from build123d import *

# Parameters (mm, degrees)
SKETCH1_W           = 15.875
SKETCH1_H           = 11.239799379
BOSS_EXTRUDE1_DEPTH = 2.54
BOSS_EXTRUDE2_REACH = 31.638
SKETCH2_W           = 1.27
SKETCH2_H           = 5.08
SKETCH2_W_2         = 3.81
SKETCH2_H_2         = 1.624267758
BOSS_EXTRUDE3_REACH = 23.94
FILLET1_R           = 0.127


with BuildPart() as part:
    # Sketch1 → Boss-Extrude1 (new body)
    with BuildSketch(Plane.XY):
        with Locations((7.9375, -19.278367991)):
            Rectangle(SKETCH1_W, SKETCH1_H)
    extrude(amount=BOSS_EXTRUDE1_DEPTH)

    # Boss-Extrude2: up to this plane
    boss_extrude2_end = Plane(origin=(1.6499976, -12.666472126, 11.206213123), z_dir=(-1.2251589112771177e-15, 0.017452406437284806, -0.9998476951563913))
    # Sketch2 → Boss-Extrude2 (add, up to the surface)
    with BuildSketch(Plane.XY.offset(2.54), mode=Mode.PRIVATE) as boss_extrude2_sk1:
        with BuildLine():
            Line((2.625, -17.673999922), (2.625, -19.753999922))
            Line((2.625, -19.753999922), (1.355, -19.753999922))
            Line((1.355, -19.753999922), (1.355, -14.673999922))
            Line((1.355, -14.673999922), (2.625, -14.673999922))
            Line((2.625, -14.673999922), (2.625, -17.273999922))
            Line((2.625, -17.273999922), (2.375, -17.273999922))
            Line((2.375, -17.273999922), (2.375, -17.473999922))
            ThreePointArc((2.375, -17.473999922), (2.433578644, -17.615421279), (2.575, -17.673999922))
            Line((2.575, -17.673999922), (2.625, -17.673999922))
        make_face()
    boss_extrude2_tool1 = split(extrude(boss_extrude2_sk1.sketch, amount=BOSS_EXTRUDE2_REACH, mode=Mode.PRIVATE), bisect_by=boss_extrude2_end, keep=Keep.BOTH, mode=Mode.PRIVATE)
    add(boss_extrude2_tool1.solids().sort_by_distance((1.982561, -17.210473, 2.54))[0])
    # Sketch2 → Boss-Extrude2 (add, up to the surface)
    with BuildSketch(Plane.XY.offset(2.54), mode=Mode.PRIVATE) as boss_extrude2_sk2:
        with Locations((10.26, -17.213999922)):
            Rectangle(SKETCH2_W, SKETCH2_H)
    boss_extrude2_tool2 = split(extrude(boss_extrude2_sk2.sketch, amount=BOSS_EXTRUDE2_REACH, mode=Mode.PRIVATE), bisect_by=boss_extrude2_end, keep=Keep.BOTH, mode=Mode.PRIVATE)
    add(boss_extrude2_tool2.solids().sort_by_distance((10.26, -17.214, 2.54))[0])
    # Sketch2 → Boss-Extrude2 (add, up to the surface)
    with BuildSketch(Plane.XY.offset(2.54), mode=Mode.PRIVATE) as boss_extrude2_sk3:
        with Locations((6.375, -24.086133801)):
            Rectangle(SKETCH2_W_2, SKETCH2_H_2)
    boss_extrude2_tool3 = split(extrude(boss_extrude2_sk3.sketch, amount=BOSS_EXTRUDE2_REACH, mode=Mode.PRIVATE), bisect_by=boss_extrude2_end, keep=Keep.BOTH, mode=Mode.PRIVATE)
    add(boss_extrude2_tool3.solids().sort_by_distance((6.375, -24.086134, 2.54))[0])

    # Boss-Extrude3: up to this face of the body (flat: up to its plane)
    boss_extrude3_end = Plane(part.part.faces().sort_by_distance((1.99, -19.753999922, 6.811249933))[0])
    # Sketch4 → Boss-Extrude3 (add, up to the picked face)
    with BuildSketch(Plane.XZ.offset(14.673999922), mode=Mode.PRIVATE) as boss_extrude3_sk1:
        Polygon((10.895, 11.082499866), (9.625, 11.082499866), (9.625, 10.790559516), (8.992585474, 11.181716662), (10.895, 14.257499866), align=None)
    boss_extrude3_tool1 = split(extrude(boss_extrude3_sk1.sketch, amount=BOSS_EXTRUDE3_REACH, mode=Mode.PRIVATE), bisect_by=boss_extrude3_end, keep=Keep.BOTH, mode=Mode.PRIVATE)
    # Sketch4 → Boss-Extrude3 (add, up to the picked face)
    with BuildSketch(Plane.XZ.offset(14.673999922), mode=Mode.PRIVATE) as boss_extrude3_sk2:
        Polygon((1.355, 11.082499866), (2.625, 11.082499866), (2.625, 10.790559516), (3.26, 11.082499866), (1.355, 14.257499866), align=None)
    boss_extrude3_tool2 = split(extrude(boss_extrude3_sk2.sketch, amount=BOSS_EXTRUDE3_REACH, mode=Mode.PRIVATE), bisect_by=boss_extrude3_end, keep=Keep.BOTH, mode=Mode.PRIVATE)
    add(boss_extrude3_tool1.solids().sort_by(Axis((10.227849, -14.674, 12.119311), (0, -1, 0)))[0])
    add(boss_extrude3_tool2.solids().sort_by(Axis((2.015179, -14.674, 12.106466), (0, -1, 0)))[0])

    # Fillet1
    fillet1_edges = [part.edges().sort_by_distance(p)[0] for p in [
        (10.895, -14.673999922, 8.398749933),
        (10.895, -19.753999922, 8.398749933),
        (1.355, -19.753999922, 8.398749933),
        (1.355, -14.673999922, 8.398749933),
        (6.375, -23.273999922, 11.021058037),
        (8.28, -24.086133801, 11.006882187),
        (6.375, -24.89826768, 10.992706338),
        (4.47, -24.086133801, 11.006882187),
        (8.992585474, -17.213999922, 11.181716662),
        (10.895, -17.213999922, 14.257499866),
        (1.355, -17.213999922, 14.257499866),
        (3.26, -17.213999922, 11.082499866),
    ]]
    fillet(fillet1_edges, radius=FILLET1_R)


solid = part.part
Input: part model. Units: mm. Frame: model coordinates. A direction names the side the tool comes from. Round coordinates to 2 decimals unless told otherwise and drop trailing zeros. Order: outer loops, then holes, each group sorted by start corner. A loop starts at its lowest first (then second) coordinate and runs counter-clockwise, first axis right, second up. Notation, with made-up numbers: (51.5, 54.25) - (63.5, 54.25) arc R15 cw to (63.5, 77.25) - close; hole circle Ø5 at (88.25, 73). An arc over 180 degrees is marked (long way). Answer as a JSON object with one key per item and string values. Group by question number.
(1) Cut plane B-B (x = 6.5). Return loops of the section in (y, z), then the cut area to 3 significant figures.
(2) Pin query (flat end, axial travel): P1, Ø1.9, axis at x = 10, z = 7, coming from the -Y side; P2, Ø3, axis at y = -23, z = 3.5, coming from the +X side (3 decimals); P3, Ø1.9, axis at x = 2.5, z = 9.5, coming from the +Y side; P4, Ø1.5, axis at y = -17, z = 10.5, coming from the +X side (3 decimals). Return the tip coordinate at first contact, or that it passes through.
(3) Cut plane C-C (y = -15.25). Return loops of the section in (x, z) (3 decimals).
(4) Material intervals for probe 1 along X at (y, z) = (-19.5, 7.5) (3 decimals); probe 2 along Z at (x, y) = (6, -20.5); probe 3 along X at (y, z) = (-17.5, 5.5) (3 decimals), sorted ascending. Write a range as from..to.
(5) Reachability of faces 1 (the face through (9.625, -17, 7)), 2 (the face through (10, -19.754, 8)), 3 (the face through (10.895, -17, 8)), 4 (the face through (4.47, -24, 7)), 5 (the face through (10, -14.674, 8)) from +Z, -Z, +X, -X, +Y, -Y: full face, straight path, thin tool, end or side. Return the list, or none.
(6) Draft query along Z for faces 6 (the face through (6, -23.274, 7)), 7 (the face through (2.4, -17.178, 12.516)), 8 (the face through (2.625, -16, 7)), 9 (the face through (8, -19, 0)). Return one class per face: released by +Z, released by -Z, zero draft, split by the parting line, or undercut.
(7) Cut plane A-A (z = 8). Return loops of the section in (x, y) (3 decimals), then the cut area to 3 significant figures.
Here are the results:
{
 "1": {"outline": "(-24.9, 0) - (-13.66, 0) - (-13.66, 2.54) - (-23.27, 2.54) - (-23.27, 10.89) arc R0.13 ccw to (-23.4, 11.02) - (-24.77, 10.99) arc R0.13 ccw to (-24.9, 10.87) - close", "area": "42.3 mm^2"},
 "2": {"P1": "stops at y = -19.75", "P2": "stops at x = 15.875", "P3": "stops at y = -14.67", "P4": "stops at x = 10.895"},
 "3": {"outline": "(0, 0) - (15.875, 0) - (15.875, 2.54) - (10.895, 2.54) - (10.895, 13.811) arc R0.127 ccw to (10.66, 13.878) - (9.059, 11.29) arc R0.127 ccw to (9.101, 11.115) - (9.625, 10.791) - (9.625, 2.54) - (2.625, 2.54) - (2.625, 10.791) - (3.131, 11.023) arc R0.127 ccw to (3.187, 11.204) - (1.591, 13.864) arc R0.127 ccw to (1.355, 13.799) - (1.355, 2.54) - (0, 2.54) - close"},
 "4": {"probe 1": "x = 1.355..2.625, 9.625..10.895", "probe 2": "z = 0..2.54", "probe 3": "x = 1.355..2.377, 9.625..10.895"},
 "5": {"face 1": "+Y, -Y", "face 2": "+Z, +X, -X, -Y", "face 3": "+Z, +X, +Y, -Y", "face 4": "+Z, -X, +Y, -Y", "face 5": "+Z, +X, -X, +Y"},
 "6": {"face 6": "zero draft", "face 7": "released by +Z", "face 8": "undercut", "face 9": "released by -Z"},
 "7": {"outline": "(1.355, -19.627) arc R0.127 ccw to (1.482, -19.754) - (2.625, -19.754) - (2.625, -17.674) - (2.575, -17.674) arc R0.2 cw to (2.375, -17.474) - (2.375, -17.274) - (2.625, -17.274) - (2.625, -14.674) - (1.482, -14.674) arc R0.127 ccw to (1.355, -14.801) - close; (4.47, -24.898) - (8.28, -24.898) - (8.28, -23.274) - (4.47, -23.274) - close; (9.625, -19.754) - (10.768, -19.754) arc R0.127 ccw to (10.895, -19.627) - (10.895, -14.801) arc R0.127 ccw to (10.768, -14.674) - (9.625, -14.674) - close", "area": "19.0 mm^2"}
}
